The listing builds one solid part. Answer for the finished solid, in the listing's coordinates (mm). Face numbers are marked on the shaded views. A direction names the side the tool comes from. Give positions to 0.01 mm unless a question says otherwise; leave off trailing zeros. Loops run counter-clockwise (first coordinate to the right, second up) from the corner with the lowest first, then second, coordinate; pieces in that order, holes last. Notation, with made-up numbers: M 29,-24.75 L 83,-24.75 A14 ccw 83,-18.75 Z; hole C 68,32.5 d6. An arc over 180 degrees is marked long. Use one line per item in the form item = value. Start each with the question number.
1. The part is cut by section B-B (x = 87). Write down the section's boundary in (y, z) (3 decimals), and give its area (3 significant figures).
2. Each of these flat-tipped pins is pushed along its axis until it touches: pin 1 Ø6 at (y, z) = (-69.5, 13) entering from -X; pin 2 Ø7.5 at (y, z) = (-264, 7.5) entering from -X; pin 3 Ø6 at (y, z) = (-140.5, 23) entering from -X. Where does it stop, or does it pass through?
3. The part is cut by section C-C (y = -232). Write down the section's boundary in (x, z).
4. Straight lines are drawn through the part: line 1 (Y direction, x = 21.5, z = 11.25); line 2 (X direction, y = -238.5, z = 21); line 3 (Y direction, x = 148, z = 23.25). For each, find the intervals that lie inside material, in ascending order. Write a range as from..to.
5. The part is cut by section D-D (y = -19.5). Write down the section's boundary in (x, z).
6. For the marked faces 5, 6, 7 and 8, determine the directions among +Z, -Z, +X, -X, +Y, -Y from which every point of the face is accessible in a straight line to the end or side of a thin tool.
7. The mould has two halves that part along Y. Classify the marked faces 1, 2, 3 and 4: released by +Y, released by -Y, zero draft, split by the parting line, or undercut.
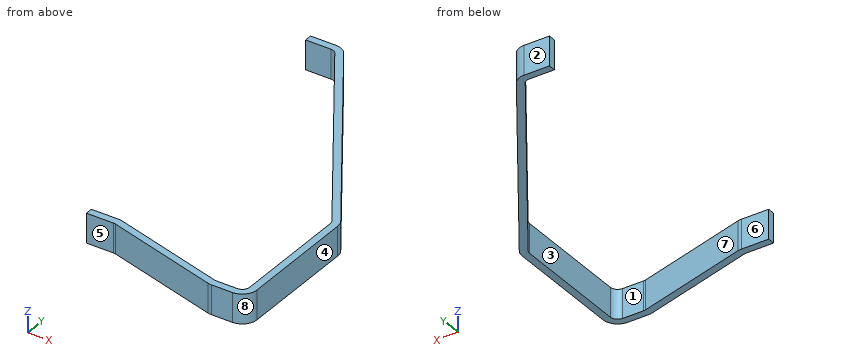
from build123d import *

# Parameters (mm, degrees)
EXTRUDE_THIN1_DEPTH = 25.4
FILLET1_R           = 6.35
FILLET2_R           = 12.7


with BuildPart() as part:
    # Sketch1 → Extrude-Thin1 (new body)
    with BuildSketch(Plane.XY):
        Polygon((0, 0), (25.4, 0), (152.4, -190.5), (152.4, -301.625), (127, -301.625), (25.4, -273.05), (0, -273.05), (0, -279.4), (24.52402436, -279.4), (126.12402436, -307.975), (158.75, -307.975), (158.75, -188.5773747), (28.798416866, 6.35), (0, 6.35), align=None)
    extrude(amount=EXTRUDE_THIN1_DEPTH)

    # Fillet1
    fillet1_edges = [part.edges().sort_by_distance(p)[0] for p in [
        (127, -301.625, 12.7),
        (152.4, -301.625, 12.7),
        (152.4, -190.5, 12.7),
        (25.4, 0, 12.7),
        (24.52402436, -279.4, 12.7),
    ]]
    fillet(fillet1_edges, radius=FILLET1_R)

    # Fillet2
    fillet2_edges = [part.edges().sort_by_distance(p)[0] for p in [
        (25.4, -273.05, 12.7),
        (28.798416866, 6.35, 12.7),
        (158.75, -188.5773747, 12.7),
        (158.75, -307.975, 12.7),
        (126.12402436, -307.975, 12.7),
    ]]
    fillet(fillet2_edges, radius=FILLET2_R)


solid = part.part
Derived:
q1.outline = M -296.971,0 L -290.375,0 L -290.375,25.4 L -296.971,25.4 Z; M -92.4,0 L -80.952,0 L -80.952,25.4 L -92.4,25.4 Z
q1.area = 458 mm2
q2.pin_1 = 69.73
q2.pin_2 = 152.4
q2.pin_3 = 117.07
q3.outline = M 152.4,0 L 158.75,0 L 158.75,25.4 L 152.4,25.4 Z
q4.line_1 = -279.4..-273.05, 0..6.35
q4.line_2 = 152.4..158.75
q4.line_3 = -307.82..-301.32, -183.9..-172.45
q5.outline = M 38.4,0 L 46.03,0 L 46.03,25.4 L 38.4,25.4 Z
q6.face_5 = +Z, -Z, -X, -Y
q6.face_6 = +Z, -Z, -X
q6.face_7 = +Z, -Z
q6.face_8 = +Z, -Z, +X, -Y
q7.face_1 = undercut
q7.face_2 = released by +Y
q7.face_3 = undercut
q7.face_4 = zero draft
